Input: part model. Units: mm. Frame: model coordinates. Face numbers are marked on the shaded views. Give positions to 0.01 mm unless a question says otherwise; leave off trailing zeros. Write each loop counter-clockwise with the first axis right and the second up, starting at its lowest first coordinate (ties: lowest second). Pieces come first, ordered by that corner, then holes. Notation, with made-up numbers: M 43,16.25 L 87,16.25 A21 ccw 87,40.25 Z; hole C -1.5,3.5 d4. An arc over 180 degrees is marked long. Use CSV: the item, a comma, the result in double quotes. Start each with the question number.
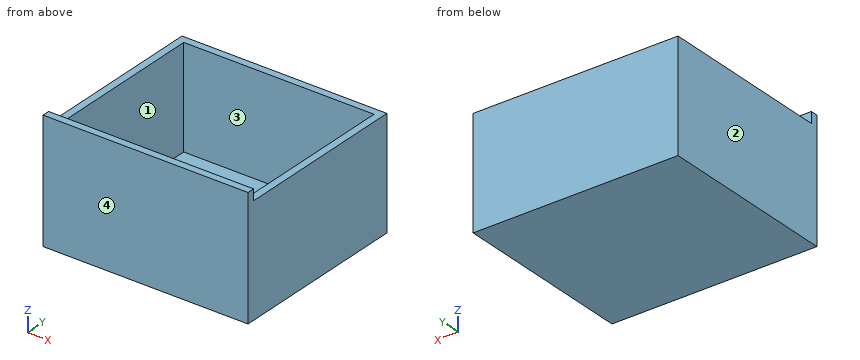
from build123d import *

# Parameters (mm, degrees)
F0_W     = 20
F0_H     = 460
F0_H_2   = 20
F0_W_2   = 520
F1_DEPTH = 300
F2_DEPTH = 330
F3_DEPTH = 25


with BuildPart() as f1:
    # F0 (on Top) → F1 (new body)
    with BuildSketch(Plane.XY):
        with Locations((-270, 0)):
            Rectangle(F0_W, F0_H)
        with Locations((-270, 240)):
            Rectangle(F0_W, F0_H_2)
        with Locations((0, 240)):
            Rectangle(F0_W_2, F0_H_2)
        with Locations((270, 240)):
            Rectangle(F0_W, F0_H_2)
        with Locations((270, 0)):
            Rectangle(F0_W, F0_H)
    extrude(amount=F1_DEPTH)

    # F0 (on Top) → F2 (join)
    with BuildSketch(Plane.XY):
        with Locations((270, -240)):
            Rectangle(F0_W, F0_H_2)
        with Locations((0, -240)):
            Rectangle(F0_W_2, F0_H_2)
        with Locations((-270, -240)):
            Rectangle(F0_W, F0_H_2)
    extrude(amount=F2_DEPTH)

    # F0 (on Top) → F3 (join)
    with BuildSketch(Plane.XY):
        Rectangle(F0_W_2, F0_H)
    extrude(amount=F3_DEPTH)


solid = f1.part
Q1. Section B-B, the plane x = 15. Return the cut outline in (y, z).
Q2. Material intervals for L1, parallel to X at y = 73, z = 53; L2, parallel to Y at x = 228.5, z = 298; L3, parallel to Z at x = 90.5, y = -189, sorted ascending. Write a range as [from, to].
Q3. Pull-direction query (X, two-part tool) for the marked faces 1, 2, 3 and 4; classes: released by +X, released by -X, zero draft, split by the parting line, or undercut.
Q4. First-contact query: pin 1 Ø1.5 at (x, y) = (-150, -91.5) entering from +Z. Flat tip, straight axial feed; report the tip coordinate or a pass-through.
Q5. Section A-A, the plane z = 230. Return the cut outline in (x, y).
Q6. Section C-C, the plane y = 84.5. Return the cut outline in (x, z).
Check result:
1,outline,"M -250,0 L 250,0 L 250,300 L 230,300 L 230,25 L -230,25 L -230,330 L -250,330 Z"
2,L1,"x = [-280, -260], [260, 280]"
2,L2,"y = [-250, -230], [230, 250]"
2,L3,"z = [0, 25]"
3,face 1,"undercut"
3,face 2,"released by -X"
3,face 3,"undercut"
3,face 4,"zero draft"
4,pin 1,"stops at z = 25"
5,outline,"M -280,-250 L 280,-250 L 280,250 L -280,250 Z; hole M -260,-230 L 260,-230 L 260,230 L -260,230 Z"
6,outline,"M -280,0 L 280,0 L 280,300 L 260,300 L 260,25 L -260,25 L -260,300 L -280,300 Z"
